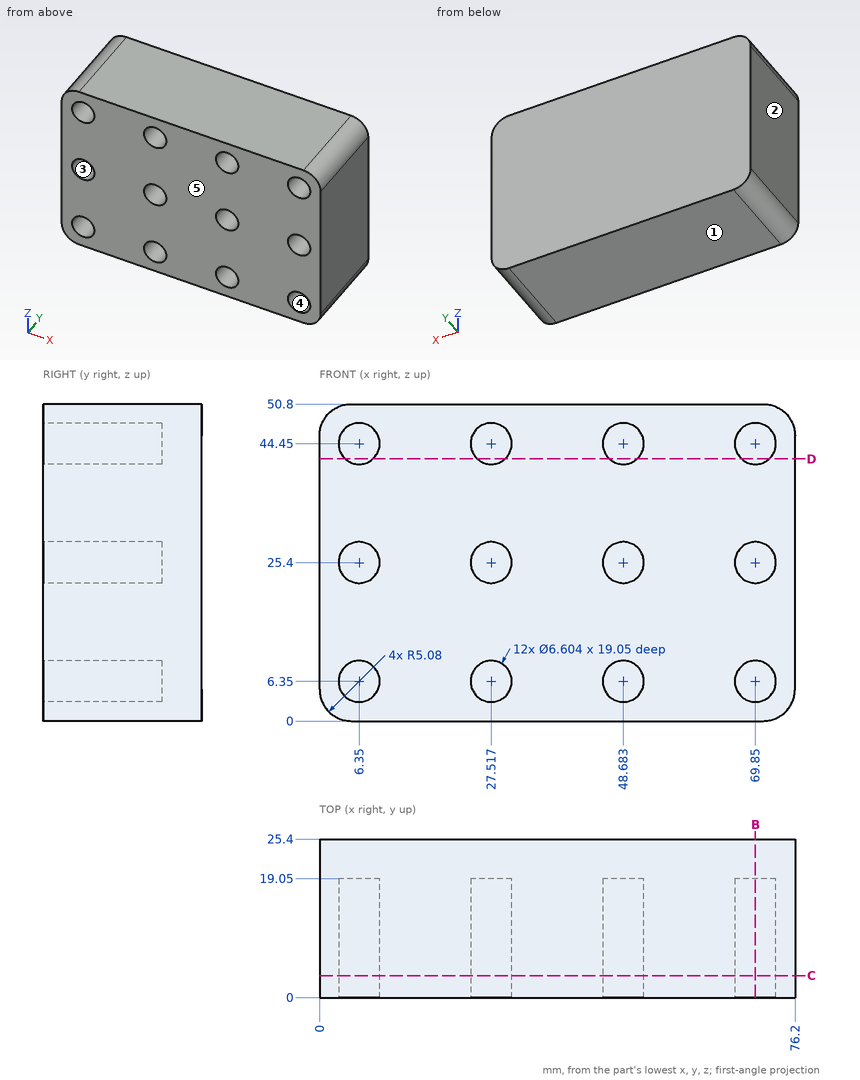
Input: dimensioned drawing with shaded views. Units: mm. Origin: part minimum x, y, z. A direction names the side the tool comes from. Give positions to 0.01 mm unless a question says otherwise; leave off trailing zeros. Order: outer loops, then holes, each group sorted by start corner. A loop starts at its lowest first (then second) coordinate and runs counter-clockwise, first axis right, second up. Notation, with made-up numbers: (40.25, -23.5) -> (47.25, -23.5) arc R22 cw to (47.25, -11.5) -> close; hole circle Ø1 at (47, 29). An arc over 180 degrees is marked (long way). Use a Markdown table: item, result.
1) Section query B-B, the plane x = 69.85. Return the cut outline in (y, z), then the cut area to 3 significant figures.
Answer list:
| item | result |
|---|---|
| outline | (0, 0) -> (25.4, 0) -> (25.4, 50.8) -> (0, 50.8) -> (0, 47.75) -> (19.05, 47.75) -> (19.05, 41.15) -> (0, 41.15) -> (0, 28.7) -> (19.05, 28.7) -> (19.05, 22.1) -> (0, 22.1) -> (0, 9.65) -> (19.05, 9.65) -> (19.05, 3.05) -> (0, 3.05) -> close |
| area | 913 mm² |
2) Contact query for a flat-ended pin moving along its axis: P1, Ø2, axis at x = 28.5, z = 46, coming from the -Y side. Output: stop coordinate, or through.
Answer list:
| item | result |
|---|---|
| P1 | y = 19.05 |
3) Mould query, pull axis X, two halves, no side actions, for the marked faces 1, 2 and 3. Classes: +X half, -X half, draft (parallel to the pull), parting line (faces both ways), or undercut.
Answer list:
| item | result |
|---|---|
| face 1 | draft |
| face 2 | -X half |
| face 3 | undercut |
4) Section query C-C, the plane y = 3.5. Count the separate pieces of the cut face and the enclosed holes in it, then the cut area to 3 significant figures.
Answer list:
| item | result |
|---|---|
| separate pieces | 1 |
| enclosed holes | 12 |
| area | 3,440 mm² |
5) Ray query, line 1 along Z through (x, y) = (70, 13.25); line 2 along Y through (x, z) = (72.5, 43.5). Return the intervals inside material, ascending. Write a range as [from, to].
Answer list:
| item | result |
|---|---|
| line 1 | [0, 3.05], [9.65, 22.1], [28.7, 41.15], [47.75, 50.8] |
| line 2 | [19.05, 25.4] |
6) Reachability of the marked faces 4 and 5 from +Z, -Z, +X, -X, +Y, -Y: full face, straight path, thin tool, end or side. Return the list, or none.
Answer list:
| item | result |
|---|---|
| face 4 | -Y |
| face 5 | +Z, -Z, +X, -X, -Y |
7) Section query D-D, the plane z = 42. Return the cut outline in (x, y), then the cut area to 3 significant figures.
Answer list:
| item | result |
|---|---|
| outline | (0, 0) -> (4.14, 0) -> (4.14, 19.05) -> (8.56, 19.05) -> (8.56, 0) -> (25.3, 0) -> (25.3, 19.05) -> (29.73, 19.05) -> (29.73, 0) -> (46.47, 0) -> (46.47, 19.05) -> (50.9, 19.05) -> (50.9, 0) -> (67.64, 0) -> (67.64, 19.05) -> (72.06, 19.05) -> (72.06, 0) -> (76.2, 0) -> (76.2, 25.4) -> (0, 25.4) -> close |
| area | 1,600 mm² |
